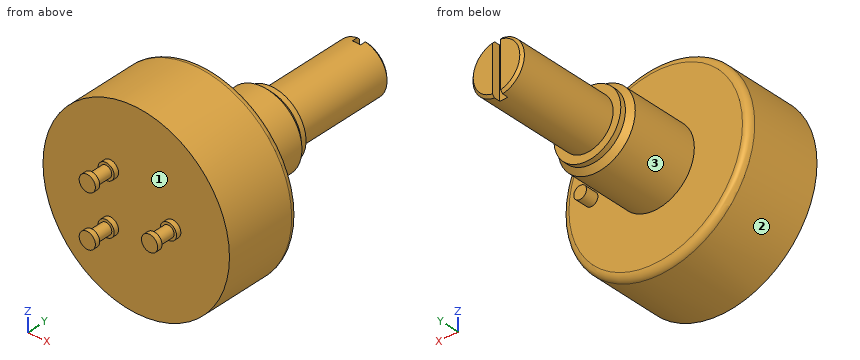
```python
from build123d import *

# Parameters (mm, degrees)
CHAMFER1_SIZE       = 0.3
SKETCH2_W           = 1
SKETCH2_H           = 6.571948564
CUT_EXTRUDE1_DEPTH  = 1
FILLET1_R           = 0.8
SKETCH3_R           = 0.785
BOSS_EXTRUDE1_DEPTH = 1.57
SKETCH4_R           = 1
BOSS_EXTRUDE2_DEPTH = 0.6
SKETCH5_R           = 0.7
BOSS_EXTRUDE3_DEPTH = 2
SKETCH6_R           = 1
BOSS_EXTRUDE4_DEPTH = 0.6


with BuildPart() as part:
    # Sketch1 → Revolve1 (revolve)
    with BuildSketch(Plane.XY):
        Polygon((0, 0), (0, 31.4), (-3.1725, 31.4), (-3.1725, 18.84), (-4.1225, 18.84), (-4.1225, 18.2), (-4.7625, 17.56), (-4.7625, 9.4), (-11.5, 9.4), (-11.5, 0), align=None)
    revolve(axis=Axis((0, 0, 0), (0, 1, 0)))

    # Chamfer1
    chamfer1_edges = [part.edges().sort_by_distance(p)[0] for p in [
        (3.1725, 31.4, 0),
    ]]
    chamfer(chamfer1_edges, length=CHAMFER1_SIZE)

    # Sketch2 → Cut-Extrude1 (cut)
    with BuildSketch(Plane(origin=(0, 31.4, 0), x_dir=(1, 0, 0), z_dir=(0, 1, 0))):
        Rectangle(SKETCH2_W, SKETCH2_H)
    extrude(amount=-CUT_EXTRUDE1_DEPTH, mode=Mode.SUBTRACT)

    # Fillet1
    fillet1_edges = [part.edges().sort_by_distance(p)[0] for p in [
        (11.5, 9.4, 0),
    ]]
    fillet(fillet1_edges, radius=FILLET1_R)

    # Sketch3 → Boss-Extrude1 (add)
    with BuildSketch(Plane(origin=(0, 9.4, 0), x_dir=(1, 0, 0), z_dir=(0, 1, 0))):
        with Locations((7.92, 0)):
            Circle(SKETCH3_R)
    extrude(amount=BOSS_EXTRUDE1_DEPTH)

    # Sketch4 → Boss-Extrude2 (add)
    with BuildSketch(Plane.XZ):
        with Locations((4.5, 0)):
            Circle(SKETCH4_R)
        with Locations((-3.181980515, 3.181980515)):
            Circle(SKETCH4_R)
        with Locations((-3.181980515, -3.181980515)):
            Circle(SKETCH4_R)
    extrude(amount=BOSS_EXTRUDE2_DEPTH)

    # Sketch5 → Boss-Extrude3 (add)
    with BuildSketch(Plane.XZ.offset(0.6)):
        with Locations((-3.181980515, 3.181980515)):
            Circle(SKETCH5_R)
        with Locations((4.5, 0)):
            Circle(SKETCH5_R)
        with Locations((-3.181980515, -3.181980515)):
            Circle(SKETCH5_R)
    extrude(amount=BOSS_EXTRUDE3_DEPTH)

    # Sketch6 → Boss-Extrude4 (add)
    with BuildSketch(Plane.XZ.offset(2.6)):
        with Locations((-3.181980515, 3.181980515)):
            Circle(SKETCH6_R)
        with Locations((4.5, 0)):
            Circle(SKETCH6_R)
        with Locations((-3.181980515, -3.181980515)):
            Circle(SKETCH6_R)
    extrude(amount=BOSS_EXTRUDE4_DEPTH)


solid = part.part
```
For this review, take the finished solid that the model builds, in its own axes (mm). Face numbers are marked on the shaded views. A direction names the side the tool comes from. Give positions to 0.01 mm unless a question says otherwise; leave off trailing zeros. Write each loop counter-clockwise with the first axis right and the second up, starting at its lowest first coordinate (ties: lowest second). Pieces come first, ordered by that corner, then holes. Notation, with made-up numbers: M 77.5,28.25 L 113.5,28.25 A13 cw 113.5,38.25 Z; hole C 0,-24.5 d10. An arc over 180 degrees is marked long. Answer as a JSON object with one key per item and string values. Group by question number.
Item 1: Consider section C-C on y = 2. Write out the cut boundary in (x, z).
Item 2: Consider section B-B on y = 10. Write out the cut boundary in (x, z) (1 decimal), plus the area to 3 significant figures.
Item 3: For probe 1 along Y at (x, z) = (0, 1.25); probe 2 along Y at (x, z) = (-8.5, -2.5); probe 3 along X at (y, z) = (28.5, -0.25), list the stretches that pass through material, from the lowest coordinate up. Write a range as [from, to].
Item 4: Consider section A-A on x = 0. Write out the cut boundary in (y, z).
Item 5: Consider section D-D on y = 21. Write out the cut boundary in (x, z) (1 decimal).
Item 6: For pin 1 Ø1.6 at (x, z) = (-3, -2.5) entering from +Y; pin 2 Ø0.5 at (x, z) = (0, -0.5) entering from +Y; pin 3 Ø12 at (x, y) = (7, 0.5) entering from -Z, all flat-tipped, find the tip position at first contact; note any pin that passes through.
Item 7: Tool access review of the marked faces 1, 2 and 3: name each direction out of +Z, -Z, +X, -X, +Y, -Y from which nothing blocks a thin tool from reaching the whole face with its end or side.
Check result:
{
 "1": {"outline": "C 0,0 d23"},
 "2": {"outline": "C 0,0 d9.5; C 7.9,0 d1.6", "area": "73.2 mm^2"},
 "3": {"probe 1": "y = [0, 30.4]", "probe 2": "y = [0, 9.4]", "probe 3": "x = [-3.16, 3.16]"},
 "4": {"outline": "M 0,-11.5 L 8.6,-11.5 A0.8 ccw 9.4,-10.7 L 9.4,-4.76 L 17.56,-4.76 L 18.2,-4.12 L 18.84,-4.12 L 18.84,-3.17 L 30.4,-3.17 L 30.4,3.17 L 18.84,3.17 L 18.84,4.12 L 18.2,4.12 L 17.56,4.76 L 9.4,4.76 L 9.4,10.7 A0.8 ccw 8.6,11.5 L 0,11.5 Z"},
 "5": {"outline": "C 0,0 d6.3"},
 "6": {"pin 1": "stops at y = 31.17", "pin 2": "stops at y = 30.4", "pin 3": "stops at z = -11.46"},
 "7": {"face 1": "-Y", "face 2": "+Y, -Y", "face 3": "+Y"}
}
